Here's how the part is built. I have some questions about the finished solid (model axes, mm). Face numbers are marked on the shaded views. A direction names the side the tool comes from. Coordinates: 2 decimals unless noted, no trailing zeros. Order: outer loops, then holes, each group sorted by start corner. A loop starts at its lowest first (then second) coordinate and runs counter-clockwise, first axis right, second up. Notation, with made-up numbers: M 40,-38.75 L 93,-38.75 A17 cw 93,-30.75 Z; hole C 80,67 d9. An arc over 180 degrees is marked long. One line per question, with ' | ' between items. Start each with the question number.
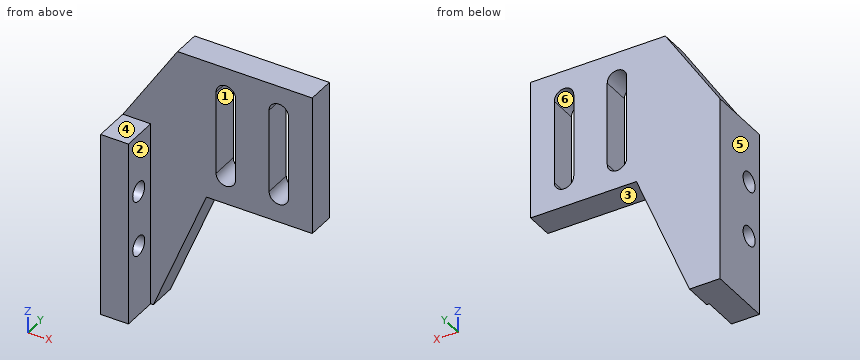
```python
from build123d import *

# Parameters (mm, degrees)
ESTRUSIONE_ESTRUSIONE8_DEPTH = 5
SCHIZZO19_W                  = 5
SCHIZZO19_H                  = 48.212351189
ESTRUSIONE_ESTRUSIONE9_DEPTH = 6.5
SCHIZZO20_R                  = 1.75
TAGLIO_ESTRUSIONE9_DEPTH     = 6
TAGLIO_ESTRUSIONE13_DEPTH    = 21
SCHIZZO26_W                  = 5
SCHIZZO26_H                  = 6.5
TAGLIO_ESTRUSIONE15_DEPTH    = 21


with BuildPart() as part:
    # Schizzo18 → Estrusione-Estrusione8 (new body)
    with BuildSketch(Plane(origin=(0, 40, 0), x_dir=(1, 0, 0), z_dir=(0, 1, 0))):
        Polygon((25, -16), (-9, -16), (-9, 32.212351189), (-3.52472969, 32.212351189), (6, 9), (25, 9), align=None)
        with BuildLine():
            Line((17.25, -11), (17.25, 4))
            ThreePointArc((17.25, 4), (19, 5.75), (20.75, 4))
            Line((20.75, 4), (20.75, -11))
            ThreePointArc((20.75, -11), (19, -12.75), (17.25, -11))
        make_face(mode=Mode.SUBTRACT)
        with BuildLine():
            Line((7.74056589, -11), (7.74056589, 4))
            ThreePointArc((7.74056589, 4), (9.49056589, 5.75), (11.24056589, 4))
            Line((11.24056589, 4), (11.24056589, -11))
            ThreePointArc((11.24056589, -11), (9.49056589, -12.75), (7.74056589, -11))
        make_face(mode=Mode.SUBTRACT)
    extrude(amount=ESTRUSIONE_ESTRUSIONE8_DEPTH)

    # Schizzo19 → Estrusione-Estrusione9 (add)
    with BuildSketch(Plane.XZ.offset(-40)):
        with Locations((-6.5, -8.106175595)):
            Rectangle(SCHIZZO19_W, SCHIZZO19_H)
    extrude(amount=ESTRUSIONE_ESTRUSIONE9_DEPTH)

    # Schizzo20 → Taglio-Estrusione9 (cut)
    with BuildSketch(Plane.ZY.offset(9)):
        with Locations((-19.5, 36.5)):
            Circle(SCHIZZO20_R)
        with Locations((-9.5, 36.5)):
            Circle(SCHIZZO20_R)
    extrude(amount=-TAGLIO_ESTRUSIONE9_DEPTH, mode=Mode.SUBTRACT)

    # Schizzo24 → Taglio-Estrusione13 (cut)
    with BuildSketch(Plane(origin=(0, 45, 0), x_dir=(1, 0, 0), z_dir=(0, 1, 0))):
        Polygon((0.805132443, -16), (-9, -0.979024983), (-9, -16), align=None)
    extrude(amount=-TAGLIO_ESTRUSIONE13_DEPTH, mode=Mode.SUBTRACT)

    # Schizzo26 → Taglio-Estrusione15 (cut)
    with BuildSketch(Plane.XY.offset(0.979024983)):
        with Locations((-6.5, 36.75)):
            Rectangle(SCHIZZO26_W, SCHIZZO26_H)
    extrude(amount=TAGLIO_ESTRUSIONE15_DEPTH, mode=Mode.SUBTRACT)


solid = part.part
```
1. Which directions (+Z, -Z, +X, -X, +Y, -Y) give clear straight access to the entire face, cutting with the end or side of a thin tool? Please do the marked faces 1, 2 and 3.
2. Imagine slicing it at A-A (x = 19). List the corners of the cut face in (y, z) for me.
3. Imagine slicing it at B-B (z = -1). List the corners of the cut face in (x, y) for me.
4. I need wall thicknesses on line 1 (Y direction, x = -7.05, z = -9.5); line 2 (X direction, y = 38.5, z = -25); line 3 (Y direction, x = 21, z = -8). Which ranges of each line are inside material? Lowest first, please.
5. Imagine slicing it at D-D (z = -19.5). List the corners of the cut face in (x, y) for me.
6. Will these pins go through, and if not, where does the flat tip stop? pin 1 (5 mm diameter, centred on y = 35, z = -18, fed in from +X); pin 2 (1.5 mm diameter, centred on y = 41.5, z = 2.5, fed in from -X); pin 3 (1.5 mm diameter, centred on x = 12, y = 42.5, fed in from -Z); pin 4 (3 mm diameter, centred on y = 36.5, z = -9.5, fed in from +X).
7. We'd pull the mould along X, two halves only. Please class the marked faces 4, 5 and 6: released by +X, released by -X, zero draft, split by the parting line, or undercut.
8. Imagine slicing it at C-C (y = 43). List the corners of the cut face in (x, z) for me, then the cut area to 3 significant figures.
Entries:
1) face 1: +Y, -Y | face 2: +Z, -Z, +X, -Y | face 3: -Z, +X, +Y, -Y
2) outline: M 40,-9 L 45,-9 L 45,-5.75 L 40,-5.75 Z; M 40,12.75 L 45,12.75 L 45,16 L 40,16 Z
3) outline: M -9,33.5 L -4,33.5 L -4,40 L 7.74,40 L 7.74,45 L -9,45 Z; M 11.24,40 L 17.25,40 L 17.25,45 L 11.24,45 Z; M 20.75,40 L 25,40 L 25,45 L 20.75,45 Z
4) line 1: 33.5 to 34.75, 38.25 to 45 | line 2: -9 to -4 | line 3: 40 to 45
5) outline: M -9,33.5 L -4,33.5 L -4,34.75 L -9,34.75 Z; M -9,38.25 L -4,38.25 L -4,40 L 1.69,40 L 1.69,45 L -9,45 Z
6) pin 1: x = -4 | pin 2: x = -8.5 | pin 3: z = -9 | pin 4: through
7) face 4: zero draft | face 5: released by -X | face 6: undercut
8) outline: M -9,-32.21 L -3.52,-32.21 L 6,-9 L 25,-9 L 25,16 L 0.81,16 L -9,0.98 Z; hole M 7.74,-4 A1.75 ccw 11.24,-4 L 11.24,11 A1.75 ccw 7.74,11 Z; hole M 17.25,-4 A1.75 ccw 20.75,-4 L 20.75,11 A1.75 ccw 17.25,11 Z | area: 890 mm²
